Source: CAD feature listing. Evaluate the final solid. Frame: model axes, mm. Face numbers are marked on the shaded views. A direction names the side the tool comes from. Round coordinates to 2 decimals unless told otherwise and drop trailing zeros. Loops run counter-clockwise (first coordinate to the right, second up) from the corner with the lowest first, then second, coordinate; pieces in that order, holes last. Notation, with made-up numbers: M -6,-30 L 52,-30 A17 cw 52,-18 Z; hole C -15,47 d11. An arc over 180 degrees is marked long. One line per item, written item: value.
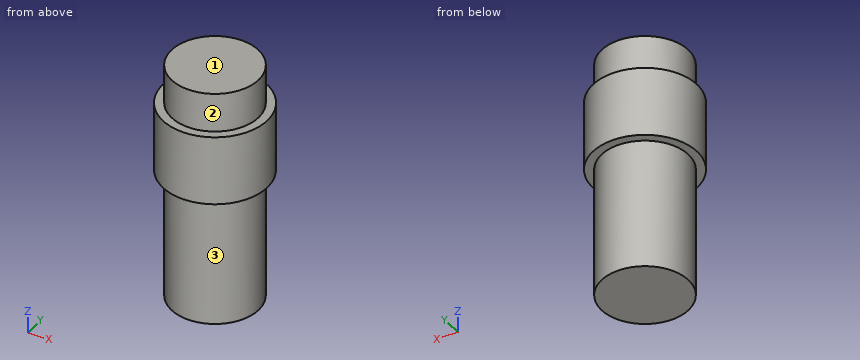
Autodesk Inventor part; units mm, degrees
ref_plane "YZ Plane" through (0, 0, 0) normal (1, 0, 0) x (0, 1, 0)
ref_plane "XZ Plane" through (0, 0, 0) normal (0, 1, 0) x (-1, 0, 0)
ref_plane "XY Plane" through (0, 0, 0) normal (0, 0, 1) x (1, 0, 0)
sketch "スケッチ1" plane through (0, 0, 0) normal (1, 0, 0) x (0, 1, 0)
  line L0 (0, 0) -> (5, 0)
  line L1 (5, 0) -> (5, 4.5)
  line L2 (5, 4.5) -> (0, 4.5)
  line L3 (0, 4.5) -> (0, 0)
  line L4 (0, 0) -> (6, 0)
  line L5 (6, 0) -> (6, -8)
  line L6 (6, -8) -> (0, -8)
  line L7 (0, -8) -> (0, 0)
  line L8 (0, -8) -> (5, -8)
  line L9 (5, -8) -> (5, -23)
  line L10 (5, -23) -> (0, -23)
  line L11 (0, -23) -> (0, -8)
  point P0 (5, 0)
  dimension "d0" = 5
  dimension "d1" = 4.5
  dimension "d2" = 6
  dimension "d3" = 8
  dimension "d4" = 15
revolve "回転1" add sketch "スケッチ1" angle 360 about axis through (0, 0, -23) along (0, 0, 1)
properties part number "出力ピン" material "鋼、炭素鋼"
1. Section query D-D (z = 1). Return the cut outline in (x, y), and give its area (3 significant figures).
Report:
outline: C 0,0 d10
area: 78.5 mm2
2. Reachability of the marked faces 1, 2 and 3 from +Z, -Z, +X, -X, +Y, -Y: full face, straight path, thin tool, end or side. Return the list, or none.
Report:
face 1: +Z, +X, -X, +Y, -Y
face 2: +Z
face 3: -Z
3. Section query A-A (x = 0). Return the cut outline in (y, z).
Report:
outline: M -6,-8 L -5,-8 L -5,-23 L 5,-23 L 5,-8 L 6,-8 L 6,0 L 5,0 L 5,4.5 L -5,4.5 L -5,0 L -6,0 Z
4. Section query C-C (z = -3.25). Return the cut outline in (x, y), and give its area (3 significant figures).
Report:
outline: C 0,0 d12
area: 113 mm2
5. Ray query, line 1 (X direction, y = -0.25, z = -16); line 2 (Y direction, x = 0.25, z = -0.5); line 3 (Y direction, x = 5, z = -5.25). Return the intervals inside material, ascending. Write a range as [from, to].
Report:
line 1: x = [-4.99, 4.99]
line 2: y = [-5.99, 5.99]
line 3: y = [-3.32, 3.32]
6. Pin query (flat end, axial travel): pin 1 (6 mm diameter, centred on x = 0, z = -16.5, fed in from +Y); pin 2 (3 mm diameter, centred on y = -5, z = -8, fed in from -X). Return the tip coordinate at first contact, or that it passes through.
Report:
pin 1: stops at y = 5
pin 2: stops at x = -4.87
